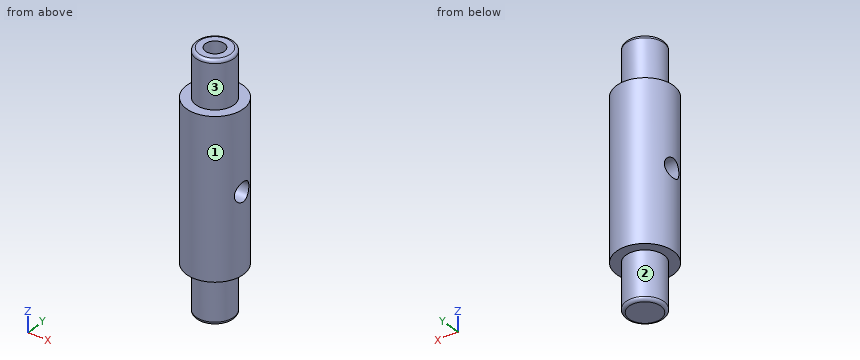
from build123d import *

# Parameters (mm, degrees)
FILLET1_R               = 1
HOLE1_D                 = 6
HOLE1_DEPTH             = 45
CUT_EXTRUDE1_DEPTH      = 42.976183724
CUT_EXTRUDE1_DEPTH_BACK = 42.976183724
SKETCH9_R               = 3


with BuildPart() as part:
    # Sketch1 → Revolve1 (revolve)
    with BuildSketch(Plane(origin=(0, 0, 0), x_dir=(0, 0, -1), z_dir=(1, 0, 0)), mode=Mode.PRIVATE) as revolve1_sk:
        Polygon((-40, 0), (-40, 6), (-25, 6), (-25, 9), (25, 9), (25, 6), (40, 6), (40, 0), align=None)
    revolve(revolve1_sk.sketch.rotate(Axis((0, 0, -40), (0, 0, 1)), 90), axis=Axis((0, 0, -40), (0, 0, 1)))

    # Fillet1
    fillet1_edges = [part.edges().sort_by_distance(p)[0] for p in [
        (6, 0, -40),
        (6, 0, 40),
    ]]
    fillet(fillet1_edges, radius=FILLET1_R)

    # Hole1
    with Locations(Plane.XY.offset(40)):
        with Locations((0, 0)):
            Hole(HOLE1_D / 2, depth=HOLE1_DEPTH)

    # Sketch9 → Cut-Extrude1 (cut, two sides: drawn at the far end of the back side and taken through both)
    with BuildSketch(Plane(origin=(0, 0, 0), x_dir=(0, 0, -1), z_dir=(1, 0, 0)).offset(-CUT_EXTRUDE1_DEPTH_BACK)):
        Circle(SKETCH9_R)
    extrude(amount=CUT_EXTRUDE1_DEPTH + CUT_EXTRUDE1_DEPTH_BACK, mode=Mode.SUBTRACT)


solid = part.part
Could you check a few things on this model? Use its own coordinates, in mm. Face numbers are marked on the shaded views. A direction names the side the tool comes from. Give positions to 0.01 mm unless a question says otherwise; leave off trailing zeros. Order: outer loops, then holes, each group sorted by start corner. A loop starts at its lowest first (then second) coordinate and runs counter-clockwise, first axis right, second up.
Item 1: If we section it at A-A, the plane y = 0: Write out the boundary of the cut face in (x, z), plus the area to 3 significant figures.
Item 2: If we section it at D-D, the plane z = 22.5: Write out the boundary of the cut face in (x, y).
Item 3: I need wall thicknesses on line 1 (Y direction, x = 0, z = -3.85); line 2 (Z direction, x = 4.25, y = 0); line 3 (X direction, y = 0.25, z = -11). Which ranges of each line are inside material? Lowest first, please.
Item 4: For the marked faces 1, 2 and 3, which set-ups out of +Z, -Z, +X, -X, +Y, -Y let a thin tool reach every point of the face, with its end or its side?
Item 5: I'm going to push flat-ended pins straight in: pin 1 (1.5 mm diameter, centred on x = 3.5, z = 8.5, fed in from +Y); pin 2 (5 mm diameter, centred on y = 0, z = 0, fed in from -X); pin 3 (2 mm diameter, centred on x = 7, y = -6, fed in from +Z); pin 4 (1 mm diameter, centred on x = -7, y = -2, fed in from -Z). Where does each tip first touch, or does it pass through?
Item 6: If we section it at B-B, the plane z = -1: Write out the boundary of the cut face in (x, y), plus the area to 3 significant figures.
Item 7: If we section it at C-C, the plane x = -7: Write out the boundary of the cut face in (y, z).
Values:
1. outline: (-9, -25) - (-6, -25) - (-6, -39) arc R1 ccw to (-5, -40) - (5, -40) arc R1 ccw to (6, -39) - (6, -25) - (9, -25) - (9, -3) - (3, -3) - (3, -5) - (-3, -5) - (-3, -3) - (-9, -3) - close; (-9, 3) - (-3, 3) - (-3, 40) - (-5, 40) arc R1 ccw to (-6, 39) - (-6, 25) - (-9, 25) - close; (3, 3) - (9, 3) - (9, 25) - (6, 25) - (6, 39) arc R1 ccw to (5, 40) - (3, 40) - close
1. area: 917 mm2
2. outline: circle Ø18 at (0, 0); hole circle Ø6 at (0, 0)
3. line 1: y = -9 to -3, 3 to 9
3. line 2: z = -40 to -3, 3 to 40
3. line 3: x = -9 to 9
4. face 1: +Z, -Z
4. face 2: -Z
4. face 3: +Z
5. pin 1: stops at y = 8.57
5. pin 2: passes through
5. pin 3: stops at z = 25
5. pin 4: stops at z = -25
6. outline: (-8.54, -2.83) arc R9 ccw to (8.54, -2.83) - (1, -2.83) arc R3 cw to (-1, -2.83) - close; (-8.54, 2.83) - (-1, 2.83) arc R3 cw to (1, 2.83) - (8.54, 2.83) arc R9 ccw to start
6. area: 154 mm2
7. outline: (-5.66, -25) - (5.66, -25) - (5.66, 25) - (-5.66, 25) - close; hole circle Ø6 at (0, 0)
